Model file for the job. Use its own axes, mm. Face numbers are marked on the shaded views. A direction names the side the tool comes from. Coordinates: 2 decimals unless noted, no trailing zeros. Write each loop counter-clockwise with the first axis right and the second up, starting at its lowest first coordinate (ties: lowest second). Pieces come first, ordered by that corner, then holes. Notation, with made-up numbers: M 69,-5.75 L 87,-5.75 A16 ccw 87,20.25 Z; hole C 56,74 d4. An arc over 180 degrees is marked long. One line per question, with ' | ' between items. Start each with the question number.
(1) Wall check: probe 1 along Z at (x, y) = (-9.25, 3.75); probe 2 along Z at (x, y) = (7.5, 10); probe 3 along Y at (x, z) = (10.5, 2). Give the ranges that are in metal, low to high.
(2) Cut at C-C (x = -9.75). Write the cut outline in (y, z).
(3) Cut at A-A (y = 11). Write the cut outline in (x, z), plus the area to 3 significant figures.
(4) Flat gauge pins, fed straight in: pin 1 Ø8 at (x, y) = (11.5, 18) entering from +Z; pin 2 Ø7.5 at (y, z) = (12, 24) entering from -X; pin 3 Ø8 at (x, z) = (10, 20) entering from +Y; pin 4 Ø1.5 at (x, z) = (8.5, 3.5) entering from +Y (3 decimals). Where does each tip first touch, or does it go through?
(5) Tool access for the marked faces 1, 2 and 3: list every direction of +Z, -Z, +X, -X, +Y, -Y with a clear straight run to the whole face (end or side of a thin tool).
(6) Cut at D-D (y = 14.5). Write the cut outline in (x, z), plus the area to 3 significant figures.
(7) Cut at B-B (z = 17.5). Write the cut outline in (x, y).
from build123d import *

# Parameters (mm, degrees)
F1_DEPTH = 15
F2_DEPTH = 5


with BuildPart() as f1:
    # F0 (on Right) → F1 (new body, symmetric)
    with BuildSketch(Plane.YZ):
        Polygon((7.5, 15), (0, 0), (30, 0), (22.5, 15), align=None)
    extrude(amount=F1_DEPTH, both=True)

    # F0 (on Right) → F2 (join, symmetric)
    with BuildSketch(Plane.YZ):
        Polygon((15, 30), (7.5, 15), (22.5, 15), align=None)
    extrude(amount=F2_DEPTH, both=True)


solid = f1.part
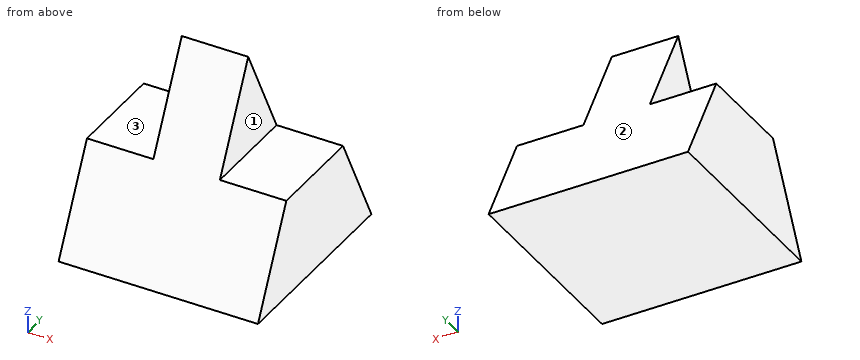
Filled in:
1) probe 1: 0 to 7.5 | probe 2: 0 to 15 | probe 3: 1 to 29
2) outline: M 0,0 L 30,0 L 22.5,15 L 7.5,15 Z
3) outline: M -15,0 L 15,0 L 15,15 L 5,15 L 5,22 L -5,22 L -5,15 L -15,15 Z | area: 520 mm²
4) pin 1: z = 15 | pin 2: x = -5 | pin 3: through | pin 4: y = 28.625
5) face 1: +Z, +X, +Y, -Y | face 2: +Z, +X, -X, +Y | face 3: +Z, -X, +Y, -Y
6) outline: M -15,0 L 15,0 L 15,15 L 5,15 L 5,29 L -5,29 L -5,15 L -15,15 Z | area: 590 mm²
7) outline: M -5,8.75 L 5,8.75 L 5,21.25 L -5,21.25 Z
